```python
from build123d import *

# Parameters (mm, degrees)
SKETCH_2_R          = 65
EXTRUDE_1_DEPTH     = 15
SKETCH_5_R          = 20
CUT_EXTRUDE_1_DEPTH = 10
SKETCH_6_R          = 3
CUT_EXTRUDE_2_DEPTH = 15


with BuildPart() as part:
    # Эскиз2 → Бобышка-Вытянуть1 (new body)
    with BuildSketch(Plane(origin=(0, 0, 0), x_dir=(1, 0, 0), z_dir=(0, 1, 0))):
        with Locations(Location((0, 0, 0), (0, 0, 270))):
            Circle(SKETCH_2_R)
    extrude(amount=EXTRUDE_1_DEPTH)

    # Эскиз5 → Вырез-Вытянуть1 (cut)
    with BuildSketch(Plane(origin=(0, 15, 0), x_dir=(1, 0, 0), z_dir=(0, 1, 0))):
        with Locations(Location((0, 0, 0), (0, 0, 270))):
            Circle(SKETCH_5_R)
    extrude(amount=-CUT_EXTRUDE_1_DEPTH, mode=Mode.SUBTRACT)

    # Эскиз6 → Вырез-Вытянуть2 (cut)
    with BuildSketch(Plane.XZ):
        with Locations(Location((0, 57.735026919, 0), (0, 0, 270))):
            Circle(SKETCH_6_R)
        with Locations(Location((-50, -28.867513459, 0), (0, 0, 270))):
            Circle(SKETCH_6_R)
        with Locations(Location((50, -28.867513459, 0), (0, 0, 270))):
            Circle(SKETCH_6_R)
    extrude(amount=-CUT_EXTRUDE_2_DEPTH, mode=Mode.SUBTRACT)


solid = part.part
```
Could you check a few things on this model? Use its own coordinates, in mm. A direction names the side the tool comes from. Round coordinates to 2 decimals unless told otherwise and drop trailing zeros. Order: outer loops, then holes, each group sorted by start corner. A loop starts at its lowest first (then second) coordinate and runs counter-clockwise, first axis right, second up. Notation, with made-up numbers: M -18.75,87.25 L 40.25,87.25 A18 ccw 40.25,115.25 Z; hole C -27.75,75 d11. An arc over 180 degrees is marked long. One line per question, with ' | ' between items. Start each with the question number.
(1) Suppose I cut it at A-A on x = 0. List the corners of the cut face in (y, z) for me.
(2) Suppose I cut it at C-C on y = 8. List the corners of the cut face in (x, z) for me.
(3) Thinking about a two-plate mould opening in X: for faces 3 (the face through (19.52, 7.4, 62)), 4 (the face through (1, 0, -1)), 5 (the face through (52.53, 7.4, -30.48)), which applies, +X half, -X half, draft (parallel to the pull), parting line (faces both ways), or undercut?
(4) For P1, Ø5.5, axis at x = 50, z = -28.87, coming from the +Y side; P2, Ø4, axis at x = 11.5, y = 13.5, coming from the -Z side; P3, Ø1.5, axis at x = 16.5, y = 9.5, coming from the +Z side; P4, Ø1, axis at x = 23.5, y = 3, coming from the +Z side, each with a flat end and sliding along its axis, tell me the tip position at first contact or that it passes through.
(5) Suppose I cut it at B-B on z = 0. List the corners of the cut face in (x, y) for me.
(6) Suppose I cut it at D-D on x = 14. List the corners of the cut face in (y, z) for me, then the cut area to 3 significant figures.
(7) Please list where these lines run through material, in increasing order: line 1 along X through (y, z) = (12, 0); line 2 along Y through (x, z) = (-4, -7); line 3 along X through (y, z) = (6.5, 2).
(8) For faces 1 (the face through (0.132, 7.395, 60.732)), 2 (the face through (0, 5, 0)), which set-ups out of +Z, -Z, +X, -X, +Y, -Y let a thin tool reach every point of the face, with its end or its side?
Geometry results:
1) outline: M 0,-65 L 15,-65 L 15,-20 L 5,-20 L 5,20 L 15,20 L 15,54.74 L 0,54.74 Z; M 0,60.74 L 15,60.74 L 15,65 L 0,65 Z
2) outline: C 0,0 d130; hole C -50,-28.87 d6; hole C 0,0 d40; hole C 0,57.74 d6; hole C 50,-28.87 d6
3) face 3: parting line | face 4: draft | face 5: undercut
4) P1: through | P2: z = -64.3 | P3: z = 63.06 | P4: z = 60.79
5) outline: M -65,0 L 65,0 L 65,15 L 20,15 L 20,5 L -20,5 L -20,15 L -65,15 Z
6) outline: M 0,-63.47 L 15,-63.47 L 15,-14.28 L 5,-14.28 L 5,14.28 L 15,14.28 L 15,63.47 L 0,63.47 Z | area: 1,620 mm²
7) line 1: -65 to -20, 20 to 65 | line 2: 0 to 5 | line 3: -64.97 to -19.9, 19.9 to 64.97
8) face 1: +Y, -Y | face 2: +Y
